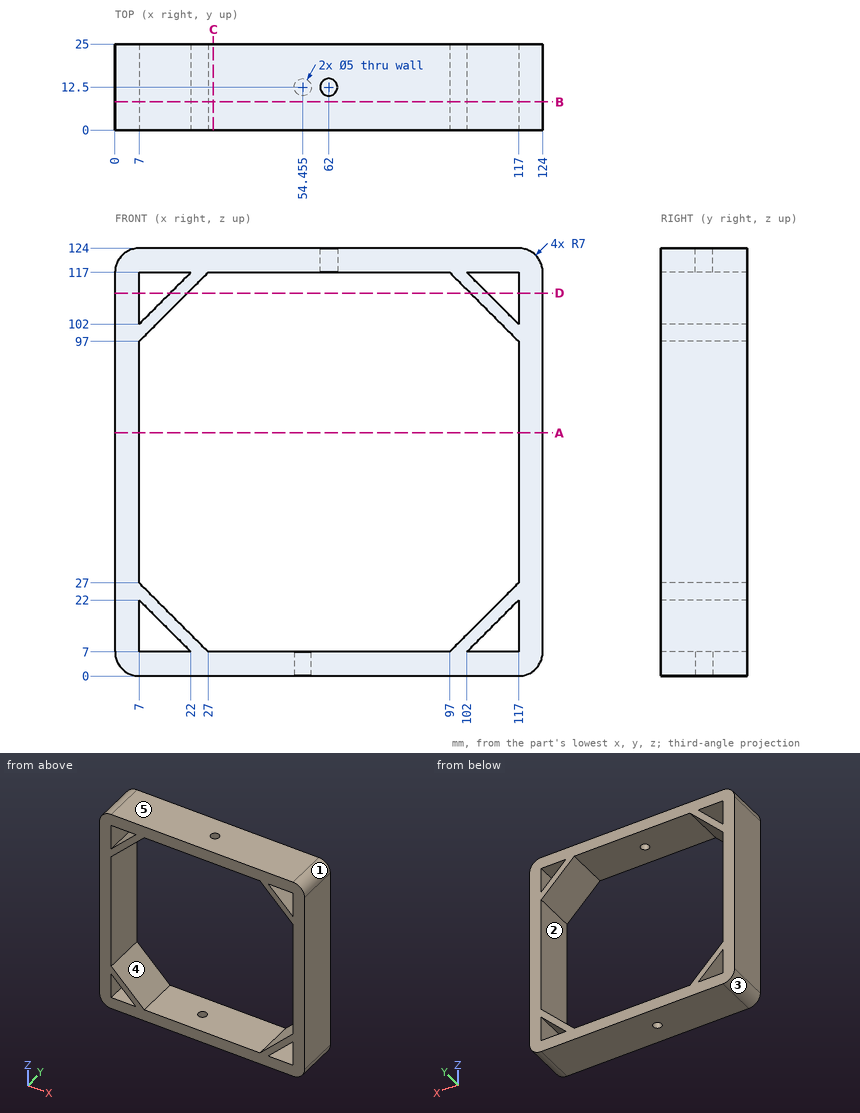
Geometry: see drawing. Coordinates: mm, zero at the bounding-box minimum. A direction names the side the tool comes from. Coordinates: 2 decimals unless noted, no trailing zeros. Loops run counter-clockwise (first coordinate to the right, second up) from the corner with the lowest first, then second, coordinate; pieces in that order, holes last. Notation, with made-up numbers: (-0.75, 29) - (39.25, 29) arc R19 ccw to (39.25, 46) - close; hole circle Ø10 at (17, -3.5). An arc over 180 degrees is marked (long way). Put each result on its own line as item: value. Start each with the question number.
Q1. Cut plane A-A, the plane z = 70.5. Return loops of the section in (x, y).
Q2. Line query: line 1 (X direction, y = 16.5, z = 52.5); line 2 (Z direction, x = 106, y = 6). Output: solid intervals per line, ascending.
Q3. Set-up query: the marked faces 1 and 2. Return all of +Z, -Z, +X, -X, +Y, -Y with unobstructed straight access to the full face (end or side cutting, diameter ignored); none if empty.
Q4. Cut plane B-B, the plane y = 8.25. Return loops of the section in (x, z), and give its area (3 significant figures).
Q5. Cut plane C-C, the plane x = 28.5. Return loops of the section in (y, z), and give its area (3 significant figures).
Q6. Pull-direction query (X, two-part tool) for the marked faces 3, 4 and 5; classes: released by +X, released by -X, zero draft, split by the parting line, or undercut.
Q7. Cut plane D-D, the plane z = 111. Return loops of the section in (x, y).
Q8. Pin query (flat end, axial travel): pin 1 Ø10 at (x, z) = (35, 16) entering from -Y. Return the tip coordinate at first contact, or that it passes through.
Filled sheet:
1. outline: (0, 0) - (7, 0) - (7, 25) - (0, 25) - close; (117, 0) - (124, 0) - (124, 25) - (117, 25) - close
2. line 1: 0 to 7, 117 to 124
2. line 2: 0 to 7, 11 to 16, 108 to 113, 117 to 124
3. face 1: +Z, +X, +Y, -Y
3. face 2: +Y, -Y
4. outline: (0, 7) arc R7 ccw to (7, 0) - (117, 0) arc R7 ccw to (124, 7) - (124, 117) arc R7 ccw to (117, 124) - (7, 124) arc R7 ccw to (0, 117) - close; hole (7, 7) - (22, 7) - (7, 22) - close; hole (7, 27) - (27, 7) - (97, 7) - (117, 27) - (117, 97) - (97, 117) - (27, 117) - (7, 97) - close; hole (7, 102) - (22, 117) - (7, 117) - close; hole (102, 7) - (117, 7) - (117, 22) - close; hole (102, 117) - (117, 102) - (117, 117) - close
4. area: 3,580 mm²
5. outline: (0, 0) - (25, 0) - (25, 7) - (0, 7) - close; (0, 117) - (25, 117) - (25, 124) - (0, 124) - close
5. area: 350 mm²
6. face 3: released by -X
6. face 4: undercut
6. face 5: zero draft
7. outline: (0, 0) - (7, 0) - (7, 25) - (0, 25) - close; (16, 0) - (21, 0) - (21, 25) - (16, 25) - close; (103, 0) - (108, 0) - (108, 25) - (103, 25) - close; (117, 0) - (124, 0) - (124, 25) - (117, 25) - close
8. pin 1: through
